Autodesk Inventor part; units mm, degrees
ref_plane "YZ Plane" through (0, 0, 0) normal (1, 0, 0) x (0, 1, 0)
ref_plane "XZ Plane" through (0, 0, 0) normal (0, 1, 0) x (-1, 0, 0)
ref_plane "XY Plane" through (0, 0, 0) normal (0, 0, 1) x (1, 0, 0)
sketch "Sketch1" plane through (0, 0, 0) normal (0, 1, 0) x (-1, 0, 0)
  line L0 (16, 0) -> (-17, 0) construction
  line L1 (0, 17) -> (0, -22.3854) construction
  circle A0 centre (0, -11.4) radius 2.5
  line L2 (18, 20) -> (-18, 20)
  line L3 (-18, 20) -> (-18, -20)
  line L4 (-18, -20) -> (18, -20)
  line L5 (18, -20) -> (18, 20)
  line L6 (18, 20) -> (-18, -20) construction
  line L7 (-18, 20) -> (18, -20) construction
  circle A1 centre (-15, 5) radius 2.5
  circle A2 centre (-15, -5) radius 2.5
  line L8 (0, 20) -> (7, 20)
  line L9 (7, 20) -> (7, -20)
  line L10 (7, -20) -> (0, -20)
  line L11 (0, -20) -> (0, 20)
  line L12 (-18, 20) -> (-8, 20)
  line L13 (-8, 20) -> (-18, 10)
  line L14 (-8, -20) -> (-18, -10)
  circle A3 centre (0, -11.4) radius 4
  circle A4 centre (-15, 5) radius 1.5183
  circle A5 centre (-15, 5) radius 4
  circle A6 centre (-15, -5) radius 4
  line L15 (-15, 1) -> (-15, -1)
  line L16 (-18, 10) -> (-31, 10)
  line L17 (-31, 10) -> (-31, -10)
  line L18 (-31, -10) -> (-18, -10)
  line L19 (-18, -10) -> (-18, 10)
  circle A7 centre (-25, -5) radius 2.5
  circle A8 centre (-25, -5) radius 4
  circle A9 centre (-25, 5) radius 2.5
  circle A10 centre (-25, 5) radius 4
  line L20 (-19, 5) -> (-21, 5)
  line L21 (-25, 1) -> (-25, -1)
  line L22 (-21, -5) -> (-19, -5)
  line L23 (-19, 5) -> (-19, -5)
  circle A11 centre (2.5, 11.4) radius 2.5
  circle A12 centre (2.5, 11.4) radius 4
  line L24 (2.5674, -8.3326) -> (2.5674, 7.4006)
  line L25 (4, -11.4) -> (4, 7.6919)
  line L26 (-11, 5) -> (-1.5, 11.4)
  line L27 (-1.5, -7.6919) -> (-11, -5)
  point P0 (0, 0)
  point P1 (-13.4817, 5)
  point P2 (-4, -11.4)
  point P3 (-15.4402, 3.5469)
  point P4 (2.5674, 8.3326)
  point P5 (0, -7.4)
  point P6 (-11, -5)
  point P7 (1.9692, -7.9183)
  point P8 (0, -15.4)
  point P9 (0, 8.2775)
  point P10 (-18, 2.3542)
  point P11 (-18, -2.3542)
  point P12 (-18, -7.6458)
  point P13 (-18, 7.6458)
  dimension "d2" = 36
  dimension "d3" = 40
  dimension "d4" = 5
  dimension "d6" = 5
  dimension "d8" = 10
  dimension "d9" = 45
  dimension "d13" = 8
  dimension "d15" = 8
  dimension "d16" = 8
  dimension "d17" = 13
  dimension "d18" = 5
  dimension "d19" = 10
  dimension "d20" = 8
  dimension "d22" = 5
  dimension "d23" = 4.5
  dimension "d24" = 8
extrude "Extrusion1" add sketch "Sketch1" along normal blind 3 contours A0 L11 A3 | A0 L11 A3 | L11 A12 L24 A3 | A3 L25 A12 L11 L2 L9 L4 | L11 L4 L14 L3 A6 L27 A3 | A12 L11 | L11 A12 | L26 A5 L3 L13 L2 L11 A12 | A6 L3 | A5 L3 | A6 L3 A5 L15 | A6 L3 | L3 L18 L17 L16 A5 L20 A10 L21 A8 L22 A6 | L3 A5 | A6 L23 A5 L3 | A8 | A10
fillet "Fillet1" radius 2 9 edges at (18, 1.5, 10) (8, 1.5, -20) (-7, 1.5, -20) (-7, 1.5, 20) (8, 1.5, 20) (31, 1.5, 10) (31, 1.5, -10) (19, 1.5, 5) (19, 1.5, -5)
properties part number "Base_3DPrint"
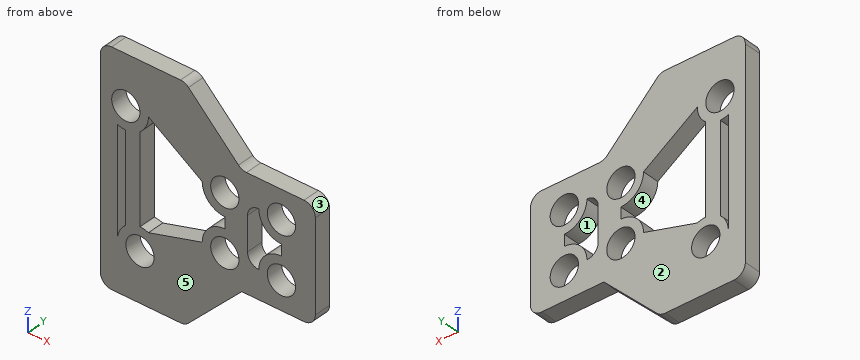
Here's how the part is built. I have some questions about the finished solid (model axes, mm). Face numbers are marked on the shaded views. A direction names the side the tool comes from. Give positions to 0.01 mm unless a question says otherwise; leave off trailing zeros. Loops run counter-clockwise (first coordinate to the right, second up) from the corner with the lowest first, then second, coordinate; pieces in that order, holes last. Notation, with made-up numbers: (-6.75, 47.25) -> (49.25, 47.25) arc R19 cw to (49.25, 79.25) -> close; hole circle Ø11 at (26.5, -36.5). An arc over 180 degrees is marked (long way). Answer as a JSON object with one key per item and string values. Group by question number.
Item 1: Thinking about a two-plate mould opening in X: for the marked faces 3, 4 and 5, which applies, pulls with the +X half, pulls with the -X half, needs draft (parallel to the pull), parting line crosses it, or undercut?
Item 2: On a 3-axis mill with a long thin cutter (end or side, diameter ignored), from which of +Z, -Z, +X, -X, +Y, -Y can I reach the whole of each face in a straight line? I mean the marked faces 1 and 2. Say none if no direction works.
Item 3: I need wall thicknesses on L1, parallel to Z at x = 16.5, y = 0.3; L2, parallel to Z at x = 24.5, y = 2.8; L3, parallel to Z at x = 17, y = 0.2. Which ranges of each line are inside material? Lowest first, please.
Item 4: Imagine slicing it at C-C on z = 17. Write out the boundary of the cut face in (x, y).
Item 5: Imagine slicing it at D-D on y = 1.6. Give the number of separate pieces and of enclosed holes in the cut face, then the cut area to 3 significant figures.
Item 6: Imagine slicing it at A-A on x = 14. Write out the boundary of the cut face in (y, z).
Item 7: Will these pins go through, and if not, where does the flat tip stop? pin 1 (6 mm diameter, centred on x = 0, z = -11.4, fed in from -Y); pin 2 (4 mm diameter, centred on x = 25, z = 5, fed in from +Y); pin 3 (1 mm diameter, centred on x = 12.5, y = 1.5, fed in from -Z); pin 4 (1.5 mm diameter, centred on x = 21.5, y = 1, fed in from +Z).
Item 8: Imagine slicing it at B-B on z = -4. Write out the boundary of the cut face in (x, y).
Answer list:
{
 "1": {"face 3": "pulls with the +X half", "face 4": "undercut", "face 5": "needs draft"},
 "2": {"face 1": "+Y, -Y", "face 2": "+Z, -Z, +X, -X, +Y"},
 "3": {"L1": "z = -11.5 to -7, -3 to 3, 7 to 11.5", "L2": "z = -10 to -7.45, -2.55 to -1.03, 1.03 to 2.55, 7.45 to 10", "L3": "z = -11 to -6.5, -3.5 to 3.5, 6.5 to 11"},
 "4": {"outline": "(-7, 0) -> (11, 0) -> (11, 3) -> (-7, 3) -> close"},
 "5": {"separate pieces": "1", "enclosed holes": "9", "area": "803 mm2"},
 "6": {"outline": "(0, -14) -> (3, -14) -> (3, -7.29) -> (0, -7.29) -> close; (0, -2.71) -> (3, -2.71) -> (3, -1.13) -> (0, -1.13) -> close; (0, 1.13) -> (3, 1.13) -> (3, 2.71) -> (0, 2.71) -> close; (0, 7.29) -> (3, 7.29) -> (3, 14) -> (0, 14) -> close"},
 "7": {"pin 1": "stops at y = 0", "pin 2": "passes through", "pin 3": "stops at z = -16", "pin 4": "stops at z = 10"},
 "8": {"outline": "(-7, 0) -> (-4, 0) -> (-4, 3) -> (-7, 3) -> close; (-2.57, 0) -> (0, 0) -> (0, 3) -> (-2.57, 3) -> close; (11.13, 0) -> (12.71, 0) -> (12.71, 3) -> (11.13, 3) -> close; (17.29, 0) -> (19.27, 0) -> (19.27, 3) -> (17.29, 3) -> close; (21.13, 0) -> (22.71, 0) -> (22.71, 3) -> (21.13, 3) -> close; (27.29, 0) -> (31, 0) -> (31, 3) -> (27.29, 3) -> close"}
}
